Read the model definition and answer for the solid it produces. Units are mm, in the model's axes. A direction names the side the tool comes from. Give positions to 0.01 mm unless a question says otherwise; leave off trailing zeros. Loops run counter-clockwise (first coordinate to the right, second up) from the corner with the lowest first, then second, coordinate; pieces in that order, holes last.
(1) Determine the mould class of faces 3 (the face through (19.5, 0, -6.8)), 4 (the face through (1.256, 90.099, -28.547)), 5 (the face through (23.4, 10.16, 8.3)) for opening direction Y: pulls with the +Y half, pulls with the -Y half, needs draft (parallel to the pull), parting line crosses it, or undercut.
(2) Straight lines are drawn through the part: probe 1 along Y at (x, z) = (-20, 15); probe 2 along X at (y, z) = (42, 0); probe 3 along X at (y, z) = (76.5, -10). For each, find the intervals that lie inside material, in ascending order.
(3) Which of the six approach directions +Z, -Z, +X, -X, +Y, -Y give full straight-line access (tool end or side, diameter ignored) to faces 1 (the face through (20.147, 48.292, -2.645)), 2 (the face through (-21.858, 47.1, 11.369))?
(4) Find section A-A, the plane x = 0. Write down the section's boundary in (y, z) (3 decimals).
(5) Find section B-B, the plane z = 0. Write down the section's boundary in (x, y) (3 decimals), then the cut area to 3 significant figures.
(6) Find section C-C, the plane y = 50. Write down the section's boundary in (x, z), then the cut area to 3 significant figures.
(7) Each of these flat-tipped pins is pushed along its axis until it touches: P1, Ø8, axis at y = 22.5, z = -7.5, coming from the +X side; P2, Ø10, axis at x = -22, y = 41.5, coming from the +Z side; P3, Ø2, axis at y = 35, z = -20.5, coming from the +X side. Where does it stop, or does it pass through?
```python
from build123d import *

# Parameters (mm, degrees)
SKETCH3_R           = 28.575
BOSS_EXTRUDE2_DEPTH = 10.16
SKETCH4_R           = 24.638
BOSS_EXTRUDE3_DEPTH = 85.09
BOSS_EXTRUDE4_START = -10.16
SKETCH5_R           = 28.575
BOSS_EXTRUDE4_DEPTH = 10.16
SKETCH6_R           = 20.32
CUT_EXTRUDE1_DEPTH  = 104.14


with BuildPart() as part:
    # Sketch3 → Boss-Extrude2 (new body)
    with BuildSketch(Plane(origin=(0, 0, 0), x_dir=(1, 0, 0), z_dir=(0, 1, 0))):
        with Locations(Location((0, 0, 0), (0, 0, 270))):
            Circle(SKETCH3_R)
    extrude(amount=BOSS_EXTRUDE2_DEPTH)

    # Sketch4 → Boss-Extrude3 (add)
    with BuildSketch(Plane(origin=(0, 10.16, 0), x_dir=(1, 0, 0), z_dir=(0, 1, 0))):
        with Locations(Location((0, 0, 0), (0, 0, 270))):
            Circle(SKETCH4_R)
    extrude(amount=BOSS_EXTRUDE3_DEPTH)

    # Sketch5 → Boss-Extrude4 (add)
    with BuildSketch(Plane(origin=(0, 95.25, 0), x_dir=(1, 0, 0), z_dir=(0, 1, 0)).offset(BOSS_EXTRUDE4_START)):
        with Locations(Location((0, 0, 0), (0, 0, 270))):
            Circle(SKETCH5_R)
    extrude(amount=BOSS_EXTRUDE4_DEPTH)

    # Sketch6 → Cut-Extrude1 (cut)
    with BuildSketch(Plane(origin=(0, 95.25, 0), x_dir=(1, 0, 0), z_dir=(0, 1, 0))):
        with Locations(Location((0, 0, 0), (0, 0, 270))):
            Circle(SKETCH6_R)
    extrude(amount=-CUT_EXTRUDE1_DEPTH, mode=Mode.SUBTRACT)


solid = part.part
```
Entries:
1. face 3: pulls with the -Y half
1. face 4: needs draft
1. face 5: undercut
2. probe 1: y = 0 to 10.16, 85.09 to 95.25
2. probe 2: x = -24.64 to -20.32, 20.32 to 24.64
2. probe 3: x = -22.52 to -17.69, 17.69 to 22.52
3. face 1: +Y, -Y
3. face 2: none
4. outline: (0, -28.575) - (10.16, -28.575) - (10.16, -24.638) - (85.09, -24.638) - (85.09, -28.575) - (95.25, -28.575) - (95.25, -20.32) - (0, -20.32) - close; (0, 20.32) - (95.25, 20.32) - (95.25, 28.575) - (85.09, 28.575) - (85.09, 24.638) - (10.16, 24.638) - (10.16, 28.575) - (0, 28.575) - close
5. outline: (-28.575, 0) - (-20.32, 0) - (-20.32, 95.25) - (-28.575, 95.25) - (-28.575, 85.09) - (-24.638, 85.09) - (-24.638, 10.16) - (-28.575, 10.16) - close; (20.32, 0) - (28.575, 0) - (28.575, 10.16) - (24.638, 10.16) - (24.638, 85.09) - (28.575, 85.09) - (28.575, 95.25) - (20.32, 95.25) - close
5. area: 983 mm2
6. outline: circle Ø49.28 at (0, 0); hole circle Ø40.64 at (0, 0)
6. area: 610 mm2
7. P1: stops at x = 24.39
7. P2: stops at z = 17.83
7. P3: stops at x = 15.06
